Geometry: see drawing. Coordinates: mm, zero at the bounding-box minimum. A direction names the side the tool comes from. Give positions to 0.01 mm unless a question says otherwise; leave off trailing zeros. Write each loop counter-clockwise with the first axis right and the second up, starting at its lowest first coordinate (ties: lowest second). Pieces come first, ordered by that corner, then holes. Notation, with made-up numbers: (39, 8) - (64, 8) arc R6 ccw to (64, 15) - close; hole circle Ø1 at (66.25, 76.5). An arc over 180 degrees is marked (long way). Use a Markdown table: item, result. Add a question column.
1. Mould query, pull axis Z, two halves, no side actions, for the marked faces 1, 2 and 3. Classes: released by +Z, released by -Z, zero draft, split by the parting line, or undercut.
2. Section query B-B, the plane x = 23.5. Return loops of the section in (y, z) (3 decimals).
3. Material intervals for probe 1 along Z at (x, y) = (32, 4.25) (3 decimals); probe 2 along Y at (x, z) = (64.5, 12.25) (3 decimals), sorted ascending.
4. Section query A-A, the plane z = 18.25. Return loops of the section in (x, y) (3 decimals), plus the area to 3 significant figures.
5. Set-up query: the marked faces 4 and 5. Return all of +Z, -Z, +X, -X, +Y, -Y with unobstructed straight access to the full face (end or side cutting, diameter ignored); none if empty.
6. Pin query (flat end, axial travel): pin 1 (11 mm diameter, centred on x = 61, y = 9.5, fed in from -Z) (3 decimals). Return the tip coordinate at first contact, or that it passes through.
7. Section query D-D, the plane x = 62. Return loops of the section in (y, z) (3 decimals).
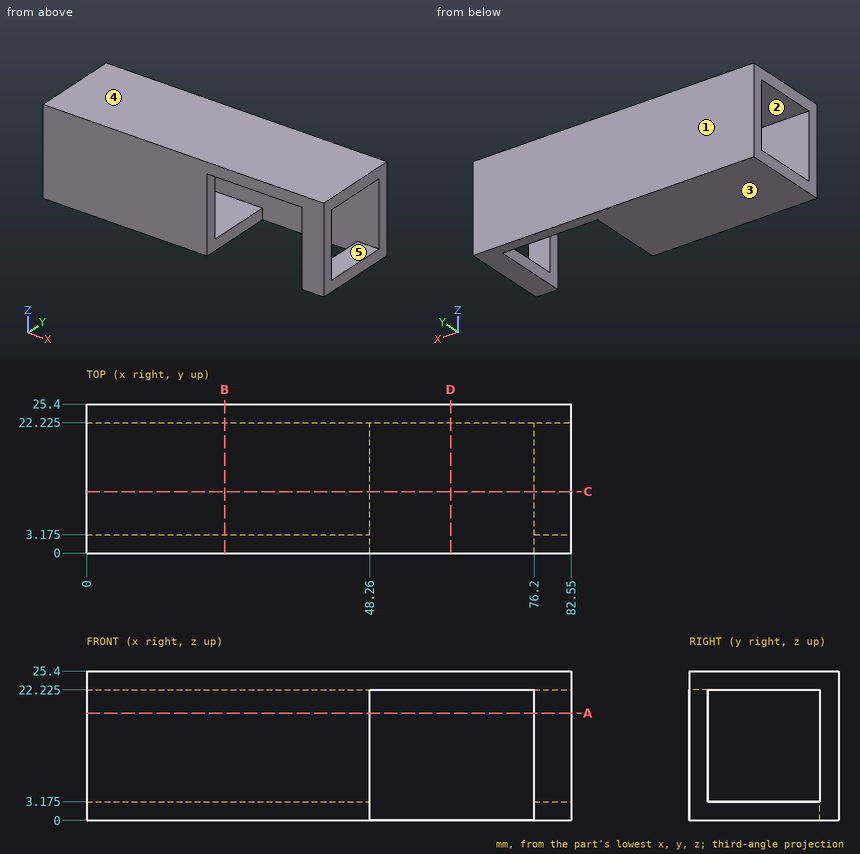
Result sheet:
| question | item | result |
|---|---|---|
| 1 | face 1 | zero draft |
| 1 | face 2 | undercut |
| 1 | face 3 | released by -Z |
| 2 | outline | (0, 0) - (25.4, 0) - (25.4, 25.4) - (0, 25.4) - close; hole (3.175, 3.175) - (22.225, 3.175) - (22.225, 22.225) - (3.175, 22.225) - close |
| 3 | probe 1 | z = 0 to 3.175, 22.225 to 25.4 |
| 3 | probe 2 | y = 22.225 to 25.4 |
| 4 | outline | (0, 0) - (48.26, 0) - (48.26, 3.175) - (0, 3.175) - close; (0, 22.225) - (82.55, 22.225) - (82.55, 25.4) - (0, 25.4) - close; (76.2, 0) - (82.55, 0) - (82.55, 3.175) - (76.2, 3.175) - close |
| 4 | area | 435 mm² |
| 5 | face 4 | +Z, +X, -X, +Y, -Y |
| 5 | face 5 | +X, -X |
| 6 | pin 1 | stops at z = 22.225 |
| 7 | outline | (0, 22.225) - (22.225, 22.225) - (22.225, 0) - (25.4, 0) - (25.4, 25.4) - (0, 25.4) - close |
